```python
from build123d import *

# Parameters (mm, degrees)
SKETCH_R        = 14.25
PAD_DEPTH       = 60
SKETCH001_W     = 28.5
SKETCH001_H     = 5.45
POCKET_DEPTH    = 60.001
SKETCH002_R     = 2
POCKET001_DEPTH = 2.4
POCKET002_DEPTH = 33.301
SKETCH004_R     = 2
POCKET003_DEPTH = 33.301
CHAMFER_SIZE2   = 2
CHAMFER_SIZE    = 2


with BuildPart() as part:
    # Sketch → Pad (new body)
    with BuildSketch(Plane.XY):
        with BuildLine():
            Line((0, 0), (0, 24.5))
            ThreePointArc((33.3, 24.5), (16.65, 41.15), (0, 24.5))
            Line((33.3, 24.5), (33.3, 0))
            Line((33.3, 0), (0, 0))
        make_face()
        with Locations((16.65, 24.5)):
            Circle(SKETCH_R, mode=Mode.SUBTRACT)
    extrude(amount=PAD_DEPTH)

    # Sketch001 (on Face7 of Pad) → Pocket (cut, through all)
    with BuildSketch(Plane.XY.offset(60)):
        with Locations((16.65, 5.125)):
            Rectangle(SKETCH001_W, SKETCH001_H)
    extrude(amount=-POCKET_DEPTH, mode=Mode.SUBTRACT)

    # Sketch002 (on Face2 of Pocket) → Pocket001 (cut)
    with BuildSketch(Plane.XZ):
        with Locations((16.65, 30)):
            Circle(SKETCH002_R)
    extrude(amount=-POCKET001_DEPTH, mode=Mode.SUBTRACT)

    # Sketch003 (on DatumPlane) → Pocket002 (cut, through all)
    with BuildSketch(Plane.YZ.offset(33.3)):
        Polygon((0, 60), (41.15, 20), (41.15, 60), align=None)
    extrude(amount=-POCKET002_DEPTH, mode=Mode.SUBTRACT)

    # Sketch004 (on Face9 of Pocket002) → Pocket003 (cut, through all)
    with BuildSketch(Plane.XZ.offset(-7.85)):
        with Locations((16.65, 10)):
            Circle(SKETCH004_R)
    extrude(amount=-POCKET003_DEPTH, mode=Mode.SUBTRACT)

    # Chamfer
    chamfer_edges = [part.edges().sort_by_distance(p)[0] for p in [
        (14.65, 41.029443, 10),
    ]]
    chamfer_side = part.faces().sort_by_distance((16.65, 41.15, 18.092345))[0]
    chamfer(chamfer_edges, length=CHAMFER_SIZE, length2=CHAMFER_SIZE2, reference=chamfer_side)


solid = part.part
```
Geometry check sheet. Reference: the model listing, model coordinates, mm. A direction names the side the tool comes from. Give positions to 0.01 mm unless a question says otherwise; leave off trailing zeros. Loops run counter-clockwise (first coordinate to the right, second up) from the corner with the lowest first, then second, coordinate; pieces in that order, holes last. Notation, with made-up numbers: M -16,-25 L -11,-25 A24 ccw -11,14 Z; hole C -4.5,61 d8. An arc over 180 degrees is marked long. Answer as CSV lines item,"result".
Item 1: Cross-section at C-C on y = 14. Record the cut outline in (x, z).
Values:
outline,"M 0,0 L 7.02,0 L 7.02,46.39 L 0,46.39 Z; M 26.28,0 L 33.3,0 L 33.3,46.39 L 26.28,46.39 Z"
Item 2: Access from +Z, -Z, +X, -X, +Y, -Y to the whole of each face (thin tool, end or side, straight path). Record for faces 5 (the cylindrical face through (17.573, 1.183, 28.226)), 6 (the cylindrical face through (18.558, 9.104, 10.601)), 7 (the flat face through (2.4, 5, 29)).
Values:
face 5,"-Y"
face 6,"+Y"
face 7,"+Z, -Z"
Item 3: Depth check by flat-ended pin: P1, Ø12, axis at x = 11.5, z = 44, coming from the +Y side; P2, Ø8.5, axis at x = 9.5, z = 23, coming from the +Y side; P3, Ø4.5, axis at x = 16.65, z = 10, coming from the +Y side. Enter the tip coordinate at first touch or a pass-through.
Values:
P1,"stops at y = 15.63"
P2,"stops at y = 40.72"
P3,"stops at y = 39.4"
Item 4: Cross-section at A-A on z = 15.5. Record the cut outline in (x, y).
Values:
outline,"M 0,0 L 33.3,0 L 33.3,24.5 A16.65 ccw 0,24.5 Z; hole M 2.4,2.4 L 30.9,2.4 L 30.9,7.85 L 2.4,7.85 Z; hole C 16.65,24.5 d28.5"
Item 5: Cross-section at B-B on x = 9. Record the cut outline in (y, z).
Values:
outline,"M 0,0 L 2.4,0 L 2.4,57.67 L 0,60 Z; M 7.85,0 L 12.48,0 L 12.48,47.87 L 7.85,52.37 Z; M 36.52,0 L 39.29,0 L 39.29,21.81 L 36.52,24.5 Z"
Item 6: Material ranges on line 1 (X direction, y = 24.5, z = 24); line 2 (Y direction, x = 7, z = 20); line 3 (Y direction, x = 11, z = 9), recorded low to high.
Values:
line 1,"x = 0 to 2.4, 30.9 to 33.3"
line 2,"y = 0 to 2.4, 7.85 to 14.01, 34.99 to 38.07"
line 3,"y = 0 to 2.4, 7.85 to 11.42, 37.58 to 40.16"
Item 7: Cross-section at D-D on z = 37. Record the cut outline in (x, y).
Values:
outline,"M 0,0 L 33.3,0 L 33.3,23.66 L 30.88,23.66 A14.25 cw 2.42,23.66 L 0,23.66 Z; hole M 2.4,2.4 L 30.9,2.4 L 30.9,7.85 L 2.4,7.85 Z"
Item 8: Release check for a two-part mould opening along Y. For faces 1 (the flat face through (17, 10, 0)), 2 (the flat face through (13, 2.4, 29)), 3 (the flat face through (30.9, 5, 29)), 4 (the flat face through (13, 0, 30)) record: pulls with the +Y half, pulls with the -Y half, needs draft (parallel to the pull), parting line crosses it, or undercut.
Values:
face 1,"needs draft"
face 2,"undercut"
face 3,"undercut"
face 4,"pulls with the -Y half"
